```python
from build123d import *

# Parameters (mm, degrees)
SKETCH2_R          = 6.925
CUT_EXTRUDE1_DEPTH = 12.580744795
SKETCH3_R          = 4.5
CUT_EXTRUDE2_DEPTH = 8.18
SKETCH4_R          = 0.925
CUT_EXTRUDE3_DEPTH = 15.400048785


with BuildPart() as part:
    # Sketch1 → Revolve1 (revolve)
    with BuildSketch(Plane.XY, mode=Mode.PRIVATE) as revolve1_sk:
        Polygon((0, 11.18), (0, 0), (1.73, 0), (1.73, 1.44), (4.69, 1.44), (4.69, 0), (6.425, 0), (6.425, 4), (4.69, 4), (4.69, 3), (4, 3), (4, 11.18), align=None)
    revolve(revolve1_sk.sketch.rotate(Axis((0, 11.18, 0), (0, -1, 0)), 90), axis=Axis((0, 11.18, 0), (0, -1, 0)))

    # Sketch2 → Cut-Extrude1 (cut, through all)
    with BuildSketch(Plane(origin=(0, 4, 0), x_dir=(1, 0, 0), z_dir=(0, 1, 0))):
        Circle(SKETCH2_R)
        Polygon((0, 6.425), (-0.735299905, 5.349704109), (-1.733444255, 6.186743571), (-2.151365885, 4.952941028), (-3.338326879, 5.489644674), (-3.407874899, 4.18884097), (-4.69562107, 4.385403945), (-4.411637422, 3.114073739), (-5.704662528, 2.955917867), (-5.088208979, 1.808349906), (-6.290615263, 1.307204884), (-5.387411354, 0.368509032), (-6.410021842, -0.438457506), (-5.287054073, -1.09866247), (-6.054026425, -2.151601508), (-4.794580179, -2.484351204), (-5.249031563, -3.70517107), (-3.946514207, -3.685786973), (-4.054740042, -4.983945043), (-2.80575333, -4.613864785), (-2.559727002, -5.893082612), (-1.456902564, -5.199753352), (-0.87487072, -6.365157203), (0, -5.4), (0.87487072, -6.365157203), (1.456902564, -5.199753352), (2.559727002, -5.893082612), (2.80575333, -4.613864785), (4.054740042, -4.983945043), (3.946514207, -3.685786973), (5.249031563, -3.70517107), (4.794580179, -2.484351204), (6.054026425, -2.151601508), (5.287054073, -1.09866247), (6.410021842, -0.438457506), (5.387411354, 0.368509032), (6.290615263, 1.307204884), (5.088208979, 1.808349906), (5.704662528, 2.955917867), (4.411637422, 3.114073739), (4.69562107, 4.385403945), (3.407874899, 4.18884097), (3.338326879, 5.489644674), (2.151365885, 4.952941028), (1.733444255, 6.186743571), (0.735299905, 5.349704109), align=None, mode=Mode.SUBTRACT)
    extrude(amount=-CUT_EXTRUDE1_DEPTH, mode=Mode.SUBTRACT)

    # Sketch3 → Cut-Extrude2 (cut)
    with BuildSketch(Plane(origin=(0, 11.18, 0), x_dir=(1, 0, 0), z_dir=(0, 1, 0))):
        Circle(SKETCH3_R)
        Polygon((0, 4), (-0.803444185, 2.472746942), (-2.351141009, 3.236067977), (-2.103444185, 1.528241656), (-3.804226065, 1.236067977), (-2.6, 0), (-3.804226065, -1.236067977), (-2.103444185, -1.528241656), (-2.351141009, -3.236067977), (-0.803444185, -2.472746942), (0, -4), (0.803444185, -2.472746942), (2.351141009, -3.236067977), (2.103444185, -1.528241656), (3.804226065, -1.236067977), (2.6, 0), (3.804226065, 1.236067977), (2.103444185, 1.528241656), (2.351141009, 3.236067977), (0.803444185, 2.472746942), align=None, mode=Mode.SUBTRACT)
    extrude(amount=-CUT_EXTRUDE2_DEPTH, mode=Mode.SUBTRACT)

    # Sketch4 → Cut-Extrude3 (cut, through all)
    with BuildSketch(Plane(origin=(0, 11.18, 0), x_dir=(1, 0, 0), z_dir=(0, 1, 0))):
        with Locations(Location((0, 0, 0), (0, 0, 270))):
            Circle(SKETCH4_R)
    extrude(amount=-CUT_EXTRUDE3_DEPTH, mode=Mode.SUBTRACT)


solid = part.part
```
Geometry: final body of the model. Coordinates: model frame, mm. A direction names the side the tool comes from. Round coordinates to 2 decimals unless told otherwise and drop trailing zeros. Write each loop counter-clockwise with the first axis right and the second up, starting at its lowest first coordinate (ties: lowest second). Pieces come first, ordered by that corner, then holes.
Item 1: Material intervals for L1, parallel to X at y = 0.7, z = 0 (3 decimals); L2, parallel to X at y = 1, z = 0.25; L3, parallel to Y at x = 0.5, z = -3.25, sorted ascending.
Item 2: Section query B-B (z = -2.25). Return loops of the section in (x, y), plus the area to 3 significant figures.
Item 3: Mould query, pull axis Z, two halves, no side actions, for faces 5 (the face through (2.226, 7.147, -2.37)), 6 (the face through (1.535, 0.73, 0.798)), 7 (the face through (-1.94, 2.03, -5.58)), 8 (the face through (-2.016, 2.028, 5.551)). Classes: +Z half, -Z half, draft (parallel to the pull), parting line (faces both ways), or undercut.
Item 4: Set-up query: faces 1 (the face through (0.373, 2.028, -5.88)), 2 (the face through (5.698, 2.028, -1.554)), 3 (the face through (2.68, 2.03, 5.26)), 4 (the face through (-5.665, 2.028, 1.618)). Return all of +Z, -Z, +X, -X, +Y, -Y with unobstructed straight access to the full face (end or side cutting, diameter ignored); none if empty.
Item 5: Section query C-C (y = 1). Give the number of separate pieces and of enclosed holes in the cut face, plus the area to 3 significant figures.
Item 6: Section query A-A (y = 10.25). Return loops of the section in (x, z) (3 decimals).
Item 7: Pin query (flat end, axial travel): P1, Ø2, axis at x = 4, y = 9.5, coming from the +Z side; P2, Ø3, axis at y = 6, z = 1.5, coming from the +X side. Return the tip coordinate at first contact, or that it passes through.
Completed:
1. L1: x = -5.854 to -4.69, -1.73 to -0.925, 0.925 to 1.73, 4.69 to 5.854
1. L2: x = -6.17 to -4.68, -1.71 to -0.89, 0.89 to 1.71, 4.68 to 6.17
1. L3: y = 1.44 to 3
2. outline: (-5.33, 0) - (-4.12, 0) - (-4.12, 1.44) - (4.12, 1.44) - (4.12, 0) - (5.33, 0) - (5.33, 4) - (4.12, 4) - (4.12, 3) - (2.21, 3) - (2.21, 11.18) - (-2.21, 11.18) - (-2.21, 3) - (-4.12, 3) - (-4.12, 4) - (-5.33, 4) - close
2. area: 58.6 mm2
3. face 5: undercut
3. face 6: undercut
3. face 7: -Z half
3. face 8: +Z half
4. face 1: -Z, +Y, -Y
4. face 2: +X, +Y, -Y
4. face 3: +Z, +Y, -Y
4. face 4: -X, +Y, -Y
5. separate pieces: 2
5. enclosed holes: 2
5. area: 46.3 mm2
6. outline: (-3.804, -1.236) - (-2.103, -1.528) - (-2.351, -3.236) - (-0.803, -2.473) - (0, -4) - (0.803, -2.473) - (2.351, -3.236) - (2.103, -1.528) - (3.804, -1.236) - (2.6, 0) - (3.804, 1.236) - (2.103, 1.528) - (2.351, 3.236) - (0.803, 2.473) - (0, 4) - (-0.803, 2.473) - (-2.351, 3.236) - (-2.103, 1.528) - (-3.804, 1.236) - (-2.6, 0) - close; hole circle Ø1.85 at (0, 0)
7. P1: stops at z = 1.37
7. P2: stops at x = 3.8
